from build123d import *

# Parameters (mm, degrees)
SKETCH1_W                                           = 150
SKETCH1_H                                           = 92.5
BOSS_EXTRUDE1_DEPTH                                 = 10
CHAMFER2_SIZE                                       = 75
CHAMFER2_SIZE2                                      = 30
CHAMFER3_SIZE                                       = 30
CHAMFER3_SIZE2                                      = 75
CBORE_FOR_M6_HEX_SOCKET_HEAD_CAP_SCREW1_D           = 6.6
CBORE_FOR_M6_HEX_SOCKET_HEAD_CAP_SCREW1_CBORE_D     = 11
CBORE_FOR_M6_HEX_SOCKET_HEAD_CAP_SCREW1_CBORE_DEPTH = 6.4
CBORE_FOR_M6_HEX_SOCKET_HEAD_CAP_SCREW2_D           = 6.6
CBORE_FOR_M6_HEX_SOCKET_HEAD_CAP_SCREW2_CBORE_D     = 11
CBORE_FOR_M6_HEX_SOCKET_HEAD_CAP_SCREW2_CBORE_DEPTH = 6.4
SKETCH11_W                                          = 150
SKETCH11_H                                          = 60
CUT_EXTRUDE1_DEPTH                                  = 3.5


with BuildPart() as part:
    # Sketch1 → Boss-Extrude1 (new, symmetric)
    with BuildSketch(Plane(origin=(0, 0, 0), x_dir=(1, 0, 0), z_dir=(0, 1, 0))):
        Rectangle(SKETCH1_W, SKETCH1_H)
    extrude(amount=BOSS_EXTRUDE1_DEPTH, both=True)

    # Chamfer2
    chamfer2_edges = [part.edges().sort_by_distance(p)[0] for p in [
        (-75, 0, 46.25),
    ]]
    chamfer2_side = [part.faces().sort_by_distance(p)[0] for p in [
        (-75, 0, 0),
    ]]
    chamfer(chamfer2_edges, length=CHAMFER2_SIZE, length2=CHAMFER2_SIZE2, reference=chamfer2_side[0])

    # Chamfer3
    chamfer3_edges = [part.edges().sort_by_distance(p)[0] for p in [
        (75, 0, 46.25),
    ]]
    chamfer3_side = [part.faces().sort_by_distance(p)[0] for p in [
        (15, 0, 46.25),
    ]]
    chamfer(chamfer3_edges, length=CHAMFER3_SIZE, length2=CHAMFER3_SIZE2, reference=chamfer3_side[0])

    # CBORE for M6 Hex Socket Head Cap Screw1 (through all)
    with Locations(Plane(origin=(0, 10, 0), x_dir=(1, 0, 0), z_dir=(0, 1, 0))):
        with Locations((-60, 31.25), (-30, 31.25), (0, 31.25), (30, 31.25), (60, 31.25)):
            CounterBoreHole(CBORE_FOR_M6_HEX_SOCKET_HEAD_CAP_SCREW1_D / 2, CBORE_FOR_M6_HEX_SOCKET_HEAD_CAP_SCREW1_CBORE_D / 2, CBORE_FOR_M6_HEX_SOCKET_HEAD_CAP_SCREW1_CBORE_DEPTH)

    # CBORE for M6 Hex Socket Head Cap Screw2 (through all)
    with Locations(Plane(origin=(0, 10, 0), x_dir=(1, 0, 0), z_dir=(0, 1, 0))):
        with Locations((-36.5, -38.25), (-36.5, -16.25), (36.5, -16.25), (36.5, -38.25)):
            CounterBoreHole(CBORE_FOR_M6_HEX_SOCKET_HEAD_CAP_SCREW2_D / 2, CBORE_FOR_M6_HEX_SOCKET_HEAD_CAP_SCREW2_CBORE_D / 2, CBORE_FOR_M6_HEX_SOCKET_HEAD_CAP_SCREW2_CBORE_DEPTH)

    # Sketch11 → Cut-Extrude1 (cut)
    with BuildSketch(Plane.XZ.offset(10)):
        with Locations((0, 26.25)):
            Rectangle(SKETCH11_W, SKETCH11_H)
    extrude(amount=-CUT_EXTRUDE1_DEPTH, mode=Mode.SUBTRACT)


solid = part.part
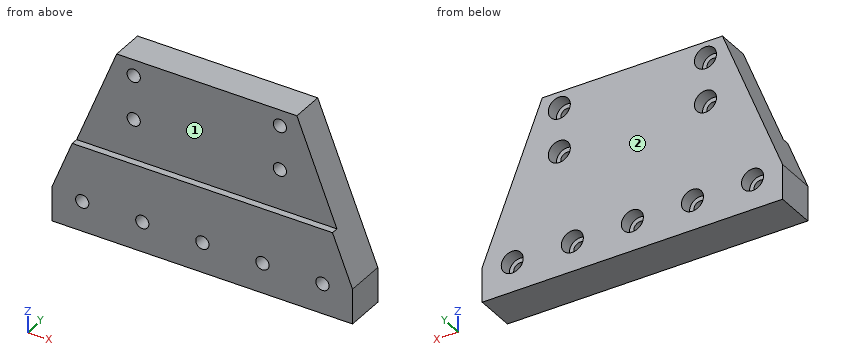
Can you work these out from the model? Positions are in its coordinate system, mm. Face numbers are marked on the shaded views. A direction names the side the tool comes from. Round coordinates to 2 decimals unless told otherwise and drop trailing zeros. Loops run counter-clockwise (first coordinate to the right, second up) from the corner with the lowest first, then second, coordinate; pieces in that order, holes last. Notation, with made-up numbers: (58, 21) - (103, 21) arc R20 ccw to (103, 30) - close; hole circle Ø4 at (-28.75, 42). An arc over 180 degrees is marked (long way). Use CSV: the item, a comma, the result in double quotes. Start each with the question number.
1) For pin 1 Ø5.5 at (x, z) = (36.5, 38.25) entering from -Y; pin 2 Ø1 at (x, y) = (-26, -7.5) entering from +Z; pin 3 Ø2 at (y, z) = (-2, -6.5) entering from +X; pin 4 Ø10.5 at (x, z) = (-30, -31.25) entering from +Y, each with a flat end and sliding along its axis, tell me the tip position at first contact or that it passes through.
2) Please list where these lines run through material, in increasing order: probe 1 along X at (y, z) = (1, -31.25); probe 2 along Z at (x, y) = (-36.5, 6); probe 3 along X at (y, z) = (7.75, -31.25). Write a range as [from, to].
3) If we section it at A-A on z = 16.25: Write out the boundary of the cut face in (x, y), plus the area to 3 significant figures.
4) If we section it at D-D on x = 23: Write out the boundary of the cut face in (y, z), plus the area to 4 significant figures.
5) If we section it at C-C on y = -4.75: Count the separate pieces of the cut face and the enclosed holes in it, plus the area to 3 significant figures.
6) For the marked faces 1 and 2, which set-ups out of +Z, -Z, +X, -X, +Y, -Y let a thin tool reach every point of the face, with its end or its side?
7) If we section it at B-B on x = 0: Write out the boundary of the cut face in (y, z), plus the area to 3 significant figures.
Geometry results:
1,pin 1,"passes through"
1,pin 2,"stops at z = -3.75"
1,pin 3,"stops at x = 66.5"
1,pin 4,"stops at y = 3.6"
2,probe 1,"x = [-75, -63.3], [-56.7, -33.3], [-26.7, -3.3], [3.3, 26.7], [33.3, 56.7], [63.3, 75]"
2,probe 2,"z = [-46.25, 10.75], [21.75, 32.75], [43.75, 46.25]"
2,probe 3,"x = [-75, -65.5], [-54.5, -35.5], [-24.5, -5.5], [5.5, 24.5], [35.5, 54.5], [65.5, 75]"
3,outline,"(-57, -6.5) - (-39.8, -6.5) - (-39.8, 3.6) - (-42, 3.6) - (-42, 10) - (-57, 10) - close; (-33.2, -6.5) - (33.2, -6.5) - (33.2, 3.6) - (31, 3.6) - (31, 10) - (-31, 10) - (-31, 3.6) - (-33.2, 3.6) - close; (39.8, -6.5) - (57, -6.5) - (57, 10) - (42, 10) - (42, 3.6) - (39.8, 3.6) - close"
3,area,"1,610 mm2"
4,outline,"(-10, -46.25) - (10, -46.25) - (10, 46.25) - (-6.5, 46.25) - (-6.5, -3.75) - (-10, -3.75) - close"
4,area,"1,675 mm2"
5,separate pieces,"1"
5,enclosed holes,"9"
5,area,"11,300 mm2"
6,face 1,"+Z, +X, -X, -Y"
6,face 2,"+Z, -Z, +X, -X, +Y"
7,outline,"(-10, -46.25) - (10, -46.25) - (10, -36.75) - (3.6, -36.75) - (3.6, -34.55) - (-10, -34.55) - close; (-10, -27.95) - (3.6, -27.95) - (3.6, -25.75) - (10, -25.75) - (10, 46.25) - (-6.5, 46.25) - (-6.5, -3.75) - (-10, -3.75) - close"
7,area,"1,510 mm2"
